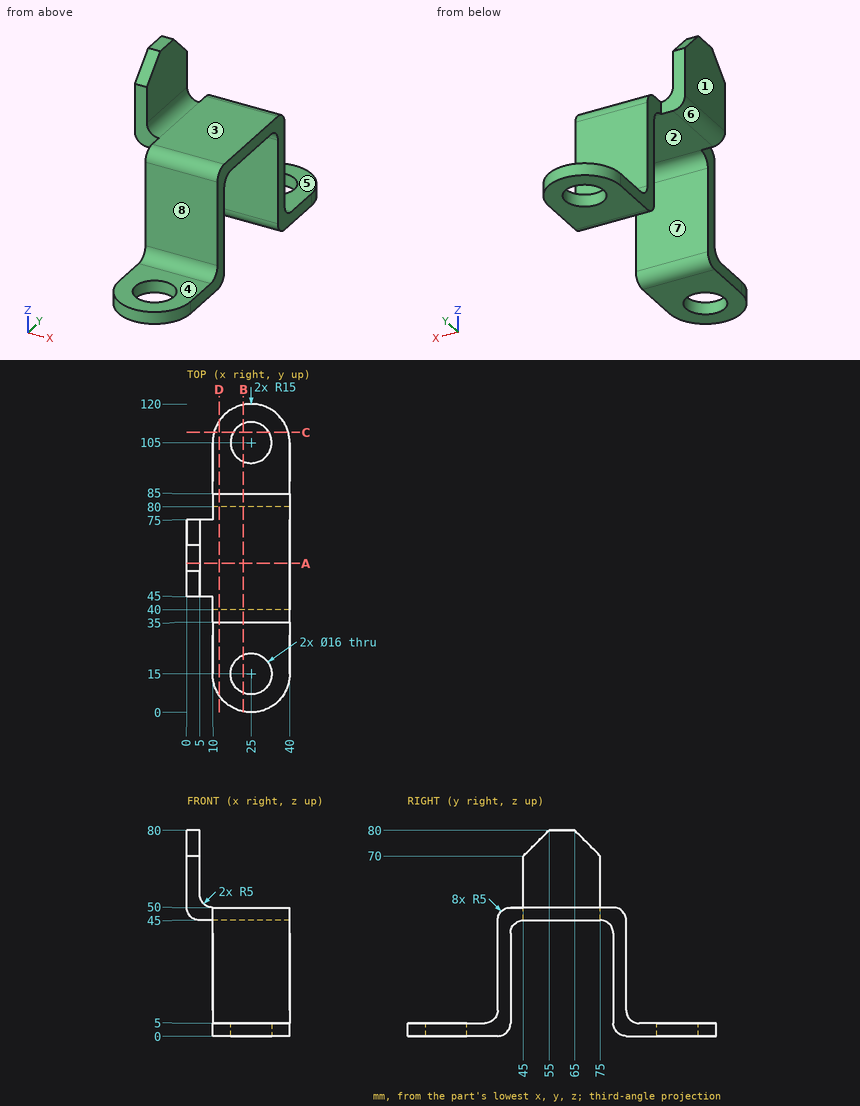
Drawing for the job (mm, zero at the part's lowest x, y, z). A direction names the side the tool comes from. Coordinates: 2 decimals unless noted, no trailing zeros. Loops run counter-clockwise (first coordinate to the right, second up) from the corner with the lowest first, then second, coordinate; pieces in that order, holes last. Notation, with made-up numbers: (17.5, 27) - (39.5, 27) arc R29 ccw to (39.5, 63) - close; hole circle Ø3 at (75, 48.25). An arc over 180 degrees is marked (long way). Use CSV: the item, a comma, the result in double quotes. Start each with the question number.
Q1. Cut at D-D, the plane x = 12.5. List the corners of the cut face in (y, z), then the cut area to 3 significant figures.
Q2. Cut at A-A, the plane y = 58. List the corners of the cut face in (x, z).
Q3. Cut at B-B, the plane x = 22. List the corners of the cut face in (y, z), then the cut area to 3 significant figures.
Q4. Drop flat-ended pins along their axis: P1, Ø10, axis at y = 40.5, z = 22.5, coming from the -X side; P2, Ø3, axis at x = 29.5, z = 33.5, coming from the +Y side; P3, Ø1, axis at x = 27.5, y = 46.5, coming from the -Z side. Give the stop position or say it passes through.
Q5. Two-plate mould, pull along Y, no slides. Class the marked faces 6, 7 and 8: +Y half, -Y half, draft (parallel to the pull), parting line (faces both ways), or undercut.
Q6. Cut at C-C, the plane y = 109. List the corners of the cut face in (x, z).
Q7. 3-axis set-ups, long thin cutter, end or side, ignore diameter. For the marked faces 1, 2, 3, 4 and 5: which of +Z, -Z, +X, -X, +Y, -Y reach the whole face in a straight line?
Q8. Probe probe 1 along X at (y, z) = (15, 3); probe 2 along Y at (x, z) = (34, 17); probe 3 along Y at (x, z) = (25, 3). List the from-to ranges inside material, lowest first. Write a range as from..to.
Here are the results:
1,outline,"(6.71, 0) - (35, 0) arc R5 ccw to (40, 5) - (40, 40) arc R5 cw to (45, 45) - (75, 45) arc R5 cw to (80, 40) - (80, 5) arc R5 ccw to (85, 0) - (113.29, 0) - (113.29, 5) - (90, 5) arc R5 cw to (85, 10) - (85, 45) arc R5 ccw to (80, 50) - (40, 50) arc R5 ccw to (35, 45) - (35, 10) arc R5 cw to (30, 5) - (6.71, 5) - close"
1,area,"983 mm2"
2,outline,"(0, 50) arc R5 ccw to (5, 45) - (40, 45) - (40, 50) - (10, 50) arc R5 cw to (5, 55) - (5, 80) - (0, 80) - close"
3,outline,"(0.3, 0) - (7.58, 0) - (7.58, 5) - (0.3, 5) - close; (22.42, 0) - (35, 0) arc R5 ccw to (40, 5) - (40, 40) arc R5 cw to (45, 45) - (75, 45) arc R5 cw to (80, 40) - (80, 5) arc R5 ccw to (85, 0) - (97.58, 0) - (97.58, 5) - (90, 5) arc R5 cw to (85, 10) - (85, 45) arc R5 ccw to (80, 50) - (40, 50) arc R5 ccw to (35, 45) - (35, 10) arc R5 cw to (30, 5) - (22.42, 5) - close; (112.42, 0) - (119.7, 0) - (119.7, 5) - (112.42, 5) - close"
3,area,"899 mm2"
4,P1,"x = 10"
4,P2,"y = 85"
4,P3,"z = 45"
5,face 6,"draft"
5,face 7,"undercut"
5,face 8,"-Y half"
6,outline,"(10.54, 0) - (18.07, 0) - (18.07, 5) - (10.54, 5) - close; (31.93, 0) - (39.46, 0) - (39.46, 5) - (31.93, 5) - close"
7,face 1,"+Z, -Z, -X, +Y, -Y"
7,face 2,"-Z, +X, -X"
7,face 3,"+Z, +X, +Y, -Y"
7,face 4,"+Z, +X, -X, -Y"
7,face 5,"+Z, +X, -X, +Y"
8,probe 1,"10..17, 33..40"
8,probe 2,"35..40, 80..85"
8,probe 3,"0..7, 23..39.58, 80.42..97, 113..120"
